```python
from build123d import *

# Parameters (mm, degrees)
SZKIC1_R                    = 10
DODANIE_WYCI_GNI_CIE2_DEPTH = 400
SZKIC3_R                    = 8
WYTNIJ_WYCI_GNI_CIE1_DEPTH  = 801
SZKIC4_R                    = 3
WYTNIJ_WYCI_GNI_CIE2_DEPTH  = 11


with BuildPart() as part:
    # Szkic1 → Dodanie-wyciągnięcie2 (new body, symmetric)
    with BuildSketch(Plane.XY):
        Circle(SZKIC1_R)
    extrude(amount=DODANIE_WYCI_GNI_CIE2_DEPTH, both=True)

    # Szkic3 → Wytnij-wyciągnięcie1 (cut, through all)
    with BuildSketch(Plane.XY.offset(400)):
        Circle(SZKIC3_R)
    extrude(amount=-WYTNIJ_WYCI_GNI_CIE1_DEPTH, mode=Mode.SUBTRACT)

    # Szkic4 → Wytnij-wyciągnięcie2 (cut, symmetric)
    with BuildSketch(Plane(origin=(0, 0, 0), x_dir=(1, 0, 0), z_dir=(0, 1, 0))):
        with Locations((0, -392.5)):
            Circle(SZKIC4_R)
    wytnij_wyci_gni_cie2 = extrude(amount=WYTNIJ_WYCI_GNI_CIE2_DEPTH, both=True, mode=Mode.SUBTRACT)

    # Lustro1: Wytnij-wyciągnięcie2 across plane
    add(wytnij_wyci_gni_cie2.mirror(Plane(origin=(0, 0, 0), x_dir=(1, 0, 0), z_dir=(0, 0, -1))), mode=Mode.SUBTRACT)


solid = part.part
```
Source: CAD feature listing. Evaluate the final solid. Frame: model axes, mm. Coordinates: 2 decimals unless noted, no trailing zeros. Loops run counter-clockwise (first coordinate to the right, second up) from the corner with the lowest first, then second, coordinate; pieces in that order, holes last. Notation, with made-up numbers: (7.5, 2) -> (12.5, 2) arc R30 cw to (12.5, 27) -> close; hole circle Ø3 at (-7.5, 52). An arc over 180 degrees is marked (long way). One line per item, written item: value. Start each with the question number.
Q1. Contact query for flat-ended pins moving along their axis: P1, Ø3.5, axis at x = 0, z = -392.5, coming from the -Y side; P2, Ø3, axis at x = -7.5, z = -207.5, coming from the -Y side; P3, Ø2, axis at x = -7, z = 252.5, coming from the +Y side; P4, Ø4, axis at x = 3.5, z = 88, coming from the -Y side. Output: stop coordinate, or through.
Q2. Line query: line 1 along Z through (x, y) = (0, -8.25); line 2 along Y through (x, z) = (1, -224); line 3 along X through (y, z) = (1.5, 61). Output: solid intervals per line, ascending.
Q3. Mould query, pull axis Y, two halves, no side actions, for faces 1 (the face through (-2.17, -9.76, 5.6)), 2 (the face through (0, 8.2, -400)), 3 (the face through (-1.73, -7.81, 5.6)). Classes: pulls with the +Y half, pulls with the -Y half, needs draft (parallel to the pull), parting line crosses it, or undercut.
Q4. Section query B-B, the plane z = -234. Return the cut outline in (x, y), and give its area (3 significant figures).
Q5. Section query A-A, the plane y = 0. Return the cut outline in (x, z).
Results:
1. P1: through
1. P2: y = -8
1. P3: y = 8
1. P4: y = -9.89
2. line 1: -400 to -395.5, -389.5 to 389.5, 395.5 to 400
2. line 2: -9.95 to -7.94, 7.94 to 9.95
2. line 3: -9.89 to -7.86, 7.86 to 9.89
3. face 1: parting line crosses it
3. face 2: needs draft
3. face 3: undercut
4. outline: circle Ø20 at (0, 0); hole circle Ø16 at (0, 0)
4. area: 113 mm^2
5. outline: (-10, -400) -> (-8, -400) -> (-8, 400) -> (-10, 400) -> close; (8, -400) -> (10, -400) -> (10, 400) -> (8, 400) -> close
